from build123d import *

# Parameters (mm, degrees)
BOSS_EXTRUDE1_DEPTH = 15.24
SKETCH3_R           = 12.7
BOSS_EXTRUDE2_DEPTH = 25.4
SKETCH4_R           = 4.3053
BOSS_EXTRUDE3_DEPTH = 10.16
EXTRUDE_THIN1_DEPTH = 2.54
SKETCH6_R           = 1.4605
CUT_EXTRUDE1_DEPTH  = 0.635


with BuildPart() as part:
    # Sketch2 → Boss-Extrude1 (new body)
    with BuildSketch(Plane(origin=(0, 0, 0), x_dir=(1, 0, 0), z_dir=(0, 1, 0))):
        Polygon((7.332348419, 12.7), (-7.332348419, 12.7), (-14.664696837, 0), (-7.332348419, -12.7), (7.332348419, -12.7), (14.664696837, 0), align=None)
    extrude(amount=BOSS_EXTRUDE1_DEPTH)

    # Sketch3 → Boss-Extrude2 (add)
    with BuildSketch(Plane(origin=(0, 15.24, 0), x_dir=(1, 0, 0), z_dir=(0, 1, 0))):
        Circle(SKETCH3_R)
    extrude(amount=BOSS_EXTRUDE2_DEPTH)

    # Sketch4 → Boss-Extrude3 (add)
    with BuildSketch(Plane.XZ):
        Circle(SKETCH4_R)
    extrude(amount=BOSS_EXTRUDE3_DEPTH)

    # Sketch5 → Extrude-Thin1 (add, symmetric)
    with BuildSketch(Plane.XY):
        Polygon((6.008182396, 40.64), (6.008182396, 50.946997676), (10.555270964, 55.659540341), (10.098307994, 56.100459659), (5.373182396, 51.203401761), (5.373182396, 40.64), align=None)
    extrude_thin1 = extrude(amount=EXTRUDE_THIN1_DEPTH, both=True)

    # Sketch6 → Cut-Extrude1 (cut)
    with BuildSketch(Plane(origin=(-22.802787707, 22.00219768, 0), x_dir=(0, 0, 1), z_dir=(-0.719626724, 0.69436113, 0))):
        with Locations((0, 43.980763894)):
            Circle(SKETCH6_R)
    cut_extrude1 = extrude(amount=-CUT_EXTRUDE1_DEPTH, mode=Mode.SUBTRACT)

    # Mirror1: Extrude-Thin1, Cut-Extrude1 across plane
    add(extrude_thin1.mirror(Plane(origin=(0, 0, 0), x_dir=(0, 0, 1), z_dir=(1, 0, 0))))
    add(cut_extrude1.mirror(Plane(origin=(0, 0, 0), x_dir=(0, 0, 1), z_dir=(1, 0, 0))), mode=Mode.SUBTRACT)


solid = part.part
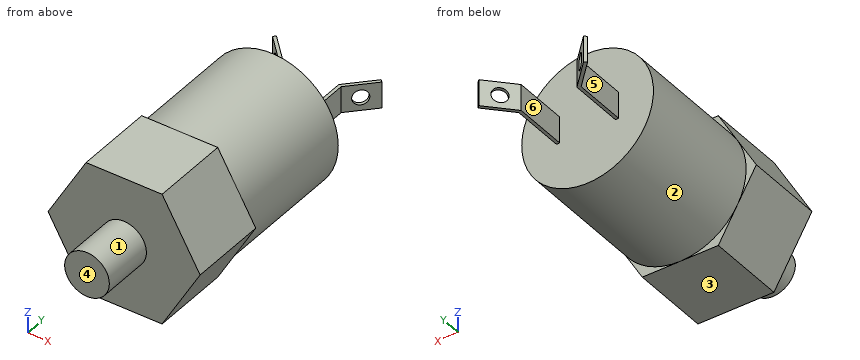
Work out the finished part from the listing and answer in its coordinate system (mm). Face numbers are marked on the shaded views. A direction names the side the tool comes from. Give positions to 0.01 mm unless a question says otherwise; leave off trailing zeros. Write each loop counter-clockwise with the first axis right and the second up, starting at its lowest first coordinate (ties: lowest second). Pieces come first, ordered by that corner, then holes. Notation, with made-up numbers: (-31.5, 84.5) - (-4.5, 84.5) arc R15 ccw to (-4.5, 109.5) - close; hole circle Ø8 at (-20, 36.5). An arc over 180 degrees is marked (long way). One line per item, written item: value. Start each with the question number.
1. Consider probe 1 along X at (y, z) = (42, -0.25); probe 2 along Y at (x, z) = (-7.75, -11.25); probe 3 along Y at (x, z) = (6.5, 5.5). Determine where each line is inside the solid, lowest interval first.
2. Find section D-D (y = 16). Write down the section's boundary in (x, z).
3. Find section C-C (y = 2). Write down the section's boundary in (x, z), then the cut area to 3 significant figures.
4. For a pull along X with two mould halves and no side action, classify the marked faces 4, 5 and 6 as +X half, -X half, draft (parallel to the pull), parting line (faces both ways), or undercut.
5. For the marked faces 1, 2 and 3, determine the directions among +Z, -Z, +X, -X, +Y, -Y from which every point of the face is accessible in a straight line to the end or side of a thin tool.
6. Given pin 1 (4 mm diameter, centred on y = 47, z = 0, fed in from +X); pin 2 (4 mm diameter, centred on x = -9, y = 50.5, fed in from +Z); pin 3 (7 mm diameter, centred on x = 5.5, z = -10, fed in from +Y); pin 4 (2.5 mm diameter, centred on y = 45.5, z = 0.5, fed in from -X), each flat-ended and moving along its own axis, determine where each tip first touches the part or whether it passes through.
7. Find section A-A (x = -3.25). Write down the section's boundary in (y, z).
8. Find section B-B (z = -5.5). Write down the section's boundary in (x, y), then the cut area to 3 significant figures.
Geometry results:
1. probe 1: -6.01 to -5.37, 5.37 to 6.01
1. probe 2: 0 to 15.24
1. probe 3: 0 to 40.64
2. outline: circle Ø25.4 at (0, 0)
3. outline: (-14.66, 0) - (-7.33, -12.7) - (7.33, -12.7) - (14.66, 0) - (7.33, 12.7) - (-7.33, 12.7) - close
3. area: 559 mm2
4. face 4: draft
4. face 5: -X half
4. face 6: undercut
5. face 1: -Y
5. face 2: +Y
5. face 3: -Z, +X, -X, +Y, -Y
6. pin 1: x = 6.01
6. pin 2: through
6. pin 3: y = 40.64
6. pin 4: x = -6.01
7. outline: (-10.16, -2.82) - (0, -2.82) - (0, -12.7) - (15.24, -12.7) - (15.24, -12.28) - (40.64, -12.28) - (40.64, 12.28) - (15.24, 12.28) - (15.24, 12.7) - (0, 12.7) - (0, 2.82) - (-10.16, 2.82) - close
8. outline: (-11.49, 0) - (11.49, 0) - (11.49, 15.24) - (11.45, 15.24) - (11.45, 40.64) - (-11.45, 40.64) - (-11.45, 15.24) - (-11.49, 15.24) - close
8. area: 932 mm2
